The listing builds one solid part. Answer for the finished solid, in the listing's coordinates (mm). A direction names the side the tool comes from. Round coordinates to 2 decimals unless told otherwise and drop trailing zeros. Write each loop counter-clockwise with the first axis right and the second up, starting at its lowest first coordinate (ties: lowest second). Pieces come first, ordered by that corner, then holes. Notation, with made-up numbers: M 79.25,-3 L 94.25,-3 A24 ccw 94.25,21 Z; hole C 87,61.5 d9. An arc over 180 degrees is marked long. One line per item, written item: value. Start each with the question number.
(1) For faces 5 (the flat face through (30, -25, 5)), 6 (the flat face through (30, 20, 25)), 7 (the flat face through (34, -20, 31)), 8 (the flat face through (20, 10, 35)), determine the directions among +Z, -Z, +X, -X, +Y, -Y from which every point of the face is accessible in a straight line to the end or side of a thin tool.
(2) Consider probe 1 along Z at (x, y) = (24.5, -8); probe 2 along X at (y, z) = (24.5, 16.5); probe 3 along X at (y, z) = (-27, 25.5). Determine where each line is inside the solid, lowest interval first.
(3) Section A-A (z = 45) is taken. Determine the outline of the cut face in (x, y), plus the area to 3 significant figures.
(4) Section B-B (y = -3) is taken. Determine the outline of the cut face in (x, z), plus the area to 3 significant figures.
(5) Section D-D (z = 16) is taken. Determine the outline of the cut face in (x, y), plus the area to 3 significant figures.
(6) Given P1, Ø10, axis at y = 16, z = 20.5, coming from the +X side; P2, Ø1.5, axis at x = 33, z = 40.5, coming from the -Y side; P3, Ø8, axis at x = 36, z = 28.5, coming from the +Y side, each flat-ended and moving along its own axis, determine where each tip first touches the part or whether it passes through.
(7) Section C-C (x = 36.5) is taken. Determine the outline of the cut face in (y, z), plus the area to 3 significant figures.
(8) For a pull along Y with two mould halves and no side action, classify faces 1 (the flat face through (30, 0, 25)), 2 (the flat face through (35, 10, 25)), 3 (the flat face through (30, -15, 25)), 4 (the flat face through (28, -8, 40)) as released by +Y, released by -Y, zero draft, split by the parting line, or undercut.
```python
from build123d import *

# Parameters (mm, degrees)
F1_DEPTH = 30
F2_W     = 10
F2_H     = 30
F3_DEPTH = 50
F4_W     = 10
F4_H     = 10
F5_DEPTH = 10
F6_W     = 10
F6_H     = 30
F7_DEPTH = 30
F8_W     = 10
F8_H     = 30
F9_DEPTH = 10


with BuildPart() as f1:
    # F0 (on Front) → F1 (new body, symmetric)
    with BuildSketch(Plane.XZ):
        Polygon((0, 50), (0, 0), (30, 0), (30, 50), (20, 50), (20, 10), (10, 10), (10, 50), align=None)
    extrude(amount=F1_DEPTH, both=True)

    # F2 (on face) → F3 (join, through all)
    with BuildSketch(Plane.XY.offset(50)):
        with Locations((35, -5)):
            Rectangle(F2_W, F2_H)
    extrude(amount=-F3_DEPTH)

    # F4 (on face) → F5 (cut)
    with BuildSketch(Plane.XZ.offset(30)):
        with Locations((25, 45)):
            Rectangle(F4_W, F4_H)
        Polygon((40, 50), (30, 50), (30, 40), (30, 0), (40, 0), align=None)
    extrude(amount=-F5_DEPTH, mode=Mode.SUBTRACT)

    # F6 (on face) → F7 (cut)
    with BuildSketch(Plane.XZ.offset(30)):
        with Locations((25, 25)):
            Rectangle(F6_W, F6_H)
    extrude(amount=-F7_DEPTH, mode=Mode.SUBTRACT)

    # F8 (on face) → F9 (cut, through all)
    with BuildSketch(Plane.YZ.offset(40)):
        with Locations((-5, 25)):
            Rectangle(F8_W, F8_H)
    extrude(amount=-F9_DEPTH, mode=Mode.SUBTRACT)


solid = f1.part
```
Recorded:
1. face 5: +Z, -Z, +X, -Y
1. face 6: +Z, -Z, +X, +Y
1. face 7: +Z, +X, -Y
1. face 8: +Z, +Y, -Y
2. probe 1: z = 0 to 10, 40 to 50
2. probe 2: x = 0 to 10, 20 to 30
2. probe 3: x = 0 to 10
3. outline: M 0,-30 L 10,-30 L 10,30 L 0,30 Z; M 20,-20 L 40,-20 L 40,10 L 30,10 L 30,30 L 20,30 Z
3. area: 1,400 mm2
4. outline: M 0,0 L 40,0 L 40,10 L 10,10 L 10,50 L 0,50 Z; M 20,40 L 40,40 L 40,50 L 20,50 Z
4. area: 1,000 mm2
5. outline: M 0,-30 L 10,-30 L 10,30 L 0,30 Z; M 20,0 L 40,0 L 40,10 L 30,10 L 30,30 L 20,30 Z; M 30,-20 L 40,-20 L 40,-10 L 30,-10 Z
5. area: 1,100 mm2
6. P1: stops at x = 30
6. P2: stops at y = -20
6. P3: stops at y = 10
7. outline: M -20,0 L 10,0 L 10,50 L -20,50 Z; hole M -10,10 L 0,10 L 0,40 L -10,40 Z
7. area: 1,200 mm2
8. face 1: undercut
8. face 2: released by +Y
8. face 3: zero draft
8. face 4: undercut
